```python
from build123d import *

# Parameters (mm, degrees)
SKETCH1_W           = 39.278818994
SKETCH1_H           = 100
SKETCH1_R           = 1.8288
SKETCH1_R_2         = 2.413
BOSS_EXTRUDE1_DEPTH = 6.35
FILLET1_R           = 3.175


with BuildPart() as part:
    # Sketch1 → Boss-Extrude1 (new body)
    # profile 1 of 2: a face of its own
    with BuildSketch(Plane(origin=(0, 0, 0), x_dir=(0, 0, -1), z_dir=(1, 0, 0))):
        with Locations((0, -53.81)):
            Rectangle(SKETCH1_W, SKETCH1_H)
        with Locations((13.4747, -100)):
            Circle(SKETCH1_R, mode=Mode.SUBTRACT)
        with Locations((-13.4747, -100)):
            Circle(SKETCH1_R, mode=Mode.SUBTRACT)
    # profile 2 of 2: a face of its own
    with BuildSketch(Plane(origin=(0, 0, 0), x_dir=(0, 0, -1), z_dir=(1, 0, 0))):
        Polygon((0, 35.468818994), (19.639409497, -3.81), (-19.639409497, -3.81), align=None)
        with Locations((13.4747, 0)):
            Circle(SKETCH1_R, mode=Mode.SUBTRACT)
        with Locations((0, 26.9494)):
            Circle(SKETCH1_R_2, mode=Mode.SUBTRACT)
        with Locations((-13.4747, 0)):
            Circle(SKETCH1_R, mode=Mode.SUBTRACT)
    extrude(amount=BOSS_EXTRUDE1_DEPTH)

    # Fillet1
    fillet1_edges = [part.edges().sort_by_distance(p)[0] for p in [
        (3.175, -3.81, 19.639409497),
        (3.175, 35.468818994, 0),
        (3.175, -3.81, -19.639409497),
        (3.175, -103.81, -19.639409497),
        (3.175, -103.81, 19.639409497),
    ]]
    fillet(fillet1_edges, radius=FILLET1_R)


solid = part.part
```
For this review, take the finished solid that the model builds, in its own axes (mm). Give positions to 0.01 mm unless a question says otherwise; leave off trailing zeros. Write each loop counter-clockwise with the first axis right and the second up, starting at its lowest first coordinate (ties: lowest second). Pieces come first, ordered by that corner, then holes. Notation, with made-up numbers: M 24,-29 L 72,-29 A33 ccw 72,9 Z; hole C 84.25,-14.75 d11. An arc over 180 degrees is marked long. Answer as a JSON object with one key per item and string values. Group by question number.
Item 1: Consider section C-C on x = 1.25. Count the separate pieces of the cut face and the enclosed holes in it, plus the area to 3 significant figures.
Item 2: For probe 1 along Y at (x, z) = (3.5, 13); probe 2 along Y at (x, z) = (5.5, 13.5); probe 3 along Y at (x, z) = (2.5, -15.5), list the stretches that pass through material, from the lowest coordinate up. Write a range as [from, to].
Item 3: Consider section B-B on y = 0. Write out the cut boundary in (x, z).
Item 4: For pin 1 Ø1.5 at (x, y) = (2, 8.5) entering from +Z, flat-tipped, find the tip position at first contact; note if it passes through.
Item 5: Draft analysis for pull direction Z (two halves, no side actions). For faces 1 (the cylindrical face through (3.13, -101.62, 12.63)), 2 (the flat face through (3.13, 13.09, 11.19)), 3 (the flat face through (6.35, -50, 0)), state which applies: +Z half, -Z half, draft (parallel to the pull), parting line (faces both ways), or undercut.
Item 6: Consider section A-A on z = 0. Write out the cut boundary in (x, y), plus the area to 3 significant figures.
Item 7: Consider section D-D on z = 6.5. Write out the cut boundary in (x, y).
Check result:
{
 "1": {"separate pieces": "1", "enclosed holes": "5", "area": "4,630 mm^2"},
 "2": {"probe 1": "y = [-103.81, -101.77], [-98.23, -1.77], [1.77, 9.47]", "probe 2": "y = [-103.81, -101.83], [-98.17, -1.83], [1.83, 8.47]", "probe 3": "y = [-103.81, 4.47]"},
 "3": {"outline": "M 0,-17.73 L 6.35,-17.73 L 6.35,-15.3 L 0,-15.3 Z; M 0,-11.65 L 6.35,-11.65 L 6.35,11.65 L 0,11.65 Z; M 0,15.3 L 6.35,15.3 L 6.35,17.73 L 0,17.73 Z"},
 "4": {"pin 1": "stops at z = 13.86"},
 "5": {"face 1": "undercut", "face 2": "+Z half", "face 3": "draft"},
 "6": {"outline": "M 0,-103.81 L 6.35,-103.81 L 6.35,24.54 L 0,24.54 Z; M 0,29.36 L 6.35,29.36 L 6.35,31.54 L 0,31.54 Z", "area": "829 mm^2"},
 "7": {"outline": "M 0,-103.81 L 6.35,-103.81 L 6.35,22.47 L 0,22.47 Z"}
}
